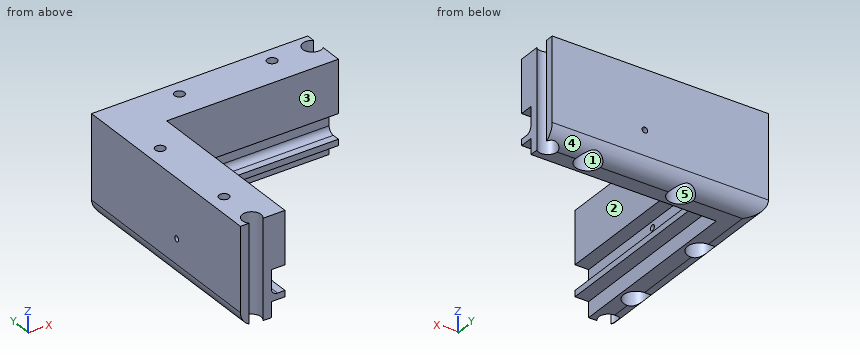
```python
from build123d import *

# Parameters (mm, degrees)
SKETCH2_W           = 18.288
SKETCH2_H           = 40.64
BOSS_EXTRUDE1_DEPTH = 88.9
SKETCH3_W           = 40.64
SKETCH3_H           = 18.288
BOSS_EXTRUDE2_DEPTH = 70.612
SKETCH4_W           = 6.35
SKETCH4_H           = 5.588
SKETCH4_W_2         = 10.16
CUT_EXTRUDE1_DEPTH  = 76.2
SKETCH5_W           = 5.588
SKETCH5_H           = 6.35
SKETCH5_H_2         = 10.16
CUT_EXTRUDE2_DEPTH  = 76.2
SKETCH6_R           = 5.08
CUT_EXTRUDE3_DEPTH  = 15.24
SKETCH7_R           = 2.032
CUT_EXTRUDE4_DEPTH  = 133.128837125
FILLET1_R           = 2.54
FILLET2_R           = 6.35
SKETCH8_R           = 3.81
CUT_EXTRUDE5_DEPTH  = 133.12883729
CUT_EXTRUDE6_REACH  = 125.941
SKETCH9_R           = 1.143
CUT_EXTRUDE7_REACH  = 125.941
SKETCH10_R          = 1.143


with BuildPart() as part:
    # Sketch2 → Boss-Extrude1 (new body)
    with BuildSketch(Plane(origin=(0, 0, 0), x_dir=(1, 0, 0), z_dir=(0, 1, 0))):
        with Locations((9.144, 20.32)):
            Rectangle(SKETCH2_W, SKETCH2_H)
    extrude(amount=BOSS_EXTRUDE1_DEPTH)

    # Sketch3 → Boss-Extrude2 (add)
    with BuildSketch(Plane(origin=(18.288, 0, 0), x_dir=(0, 0, -1), z_dir=(1, 0, 0))):
        with Locations((20.32, 79.756)):
            Rectangle(SKETCH3_W, SKETCH3_H)
    extrude(amount=BOSS_EXTRUDE2_DEPTH)

    # Sketch4 → Cut-Extrude1 (cut)
    with BuildSketch(Plane(origin=(88.9, 0, 0), x_dir=(0, 0, -1), z_dir=(1, 0, 0))):
        with Locations((37.465, 73.406)):
            Rectangle(SKETCH4_W, SKETCH4_H)
        with Locations((26.67, 73.406)):
            Rectangle(SKETCH4_W_2, SKETCH4_H)
    extrude(amount=-CUT_EXTRUDE1_DEPTH, mode=Mode.SUBTRACT)

    # Sketch5 → Cut-Extrude2 (cut)
    with BuildSketch(Plane.XZ):
        with Locations((15.494, -37.465)):
            Rectangle(SKETCH5_W, SKETCH5_H)
        with Locations((15.494, -26.67)):
            Rectangle(SKETCH5_W, SKETCH5_H_2)
    extrude(amount=-CUT_EXTRUDE2_DEPTH, mode=Mode.SUBTRACT)

    # Sketch6 → Cut-Extrude3 (cut)
    with BuildSketch(Plane(origin=(0, 0, -40.64), x_dir=(-1, 0, 0), z_dir=(0, 0, -1))):
        with Locations((-6.35, 19.05)):
            Circle(SKETCH6_R)
        with Locations((-6.35, 57.15)):
            Circle(SKETCH6_R)
        with Locations((-31.75, 82.55)):
            Circle(SKETCH6_R)
        with Locations((-69.85, 82.55)):
            Circle(SKETCH6_R)
    extrude(amount=-CUT_EXTRUDE3_DEPTH, mode=Mode.SUBTRACT)

    # Sketch7 → Cut-Extrude4 (cut, through all)
    with BuildSketch(Plane(origin=(0, 0, -40.64), x_dir=(-1, 0, 0), z_dir=(0, 0, -1))):
        with Locations((-69.85, 82.55)):
            Circle(SKETCH7_R)
        with Locations((-6.35, 57.15)):
            Circle(SKETCH7_R)
        with Locations((-31.75, 82.55)):
            Circle(SKETCH7_R)
        with Locations((-6.35, 19.05)):
            Circle(SKETCH7_R)
    extrude(amount=-CUT_EXTRUDE4_DEPTH, mode=Mode.SUBTRACT)

    # Fillet1
    fillet1_edges = [part.edges().sort_by_distance(p)[0] for p in [
        (12.7, 38.1, -31.75),
        (50.8, 76.2, -31.75),
    ]]
    fillet(fillet1_edges, radius=FILLET1_R)

    # Fillet2
    # the kernel refuses this fillet: 6.35 mm, written as the material it takes off along each edge
    with BuildSketch(Plane(origin=(104.775, 88.9, -40.64), x_dir=(0, -1, 0), z_dir=(-1, 0, 0))) as fillet2_piece_1:
        with BuildLine():
            CenterArc((FILLET2_R, FILLET2_R), FILLET2_R, 180, 90)
            Line((0, FILLET2_R), (0, 0))
            Line((0, 0), (FILLET2_R, 0))
        make_face()
    extrude(amount=120.65, mode=Mode.SUBTRACT)
    with BuildSketch(Plane(origin=(0, -15.875, -40.64), x_dir=(1, 0, 0), z_dir=(0, 1, 0))) as fillet2_piece_2:
        with BuildLine():
            CenterArc((FILLET2_R, -FILLET2_R), FILLET2_R, 90, 90)
            Line((0, -FILLET2_R), (0, 0))
            Line((0, 0), (FILLET2_R, 0))
        make_face()
    extrude(amount=120.65, mode=Mode.SUBTRACT)

    # Sketch8 → Cut-Extrude5 (cut, through all)
    with BuildSketch(Plane.XY):
        with Locations((6.35, 2.54)):
            Circle(SKETCH8_R)
        with Locations((86.36, 82.55)):
            Circle(SKETCH8_R)
    extrude(amount=-CUT_EXTRUDE5_DEPTH, mode=Mode.SUBTRACT)

    # Sketch9 → Cut-Extrude6 (cut, up to next)
    with BuildSketch(Plane.XZ.offset(-76.2), mode=Mode.PRIVATE) as cut_extrude6_sk1:
        with Locations((50.8, -24.13)):
            Circle(SKETCH9_R)
    cut_extrude6_tool1 = extrude(cut_extrude6_sk1.sketch, amount=-CUT_EXTRUDE6_REACH, mode=Mode.PRIVATE) & part.part
    add(cut_extrude6_tool1.solids().sort_by_distance((50.8, 76.2, -24.13))[0], mode=Mode.SUBTRACT)

    # Sketch10 → Cut-Extrude7 (cut, up to next)
    with BuildSketch(Plane(origin=(12.7, 0, 0), x_dir=(0, 0, -1), z_dir=(1, 0, 0)), mode=Mode.PRIVATE) as cut_extrude7_sk1:
        with Locations((24.13, 38.1)):
            Circle(SKETCH10_R)
    cut_extrude7_tool1 = extrude(cut_extrude7_sk1.sketch, amount=-CUT_EXTRUDE7_REACH, mode=Mode.PRIVATE) & part.part
    add(cut_extrude7_tool1.solids().sort_by_distance((12.7, 38.1, -24.13))[0], mode=Mode.SUBTRACT)


solid = part.part
```
Read the model definition and answer for the solid it produces. Units are mm, in the model's axes. Face numbers are marked on the shaded views. A direction names the side the tool comes from. Give positions to 0.01 mm unless a question says otherwise; leave off trailing zeros. Order: outer loops, then holes, each group sorted by start corner. A loop starts at its lowest first (then second) coordinate and runs counter-clockwise, first axis right, second up. Notation, with made-up numbers: (76, 63.5) -> (119, 63.5) arc R10 ccw to (119, 79.5) -> close; hole circle Ø8 at (-39, 54.5). An arc over 180 degrees is marked (long way). Write item = value, one per line.
1. Straight lines are drawn through the part: line 1 along X through (y, z) = (57.15, -32.5); line 2 along Z through (x, y) = (16, 48.5); line 3 along X through (y, z) = (84, -25.5). For each, find the intervals that lie inside material, in ascending order.
Numbers:
line_1 = 0 to 1.27, 11.43 to 18.29
line_2 = -34.29 to -31.75, -21.59 to 0
line_3 = 0 to 26.88, 36.62 to 64.98, 74.72 to 82.84
2. A cutting plane is placed at A-A, the plane z = -24.13. Write down the section's boundary in (x, y), and give its area (3 significant figures).
Numbers:
outline = (0, 0) -> (3.51, 0) arc R3.81 cw (long way) to (9.19, 0) -> (12.7, 0) -> (12.7, 36.96) -> (0, 36.96) -> close; (0, 39.24) -> (12.7, 39.24) -> (12.7, 76.2) -> (49.66, 76.2) -> (49.66, 88.9) -> (0, 88.9) -> close; (51.94, 76.2) -> (88.9, 76.2) -> (88.9, 79.71) arc R3.81 cw (long way) to (88.9, 85.39) -> (88.9, 88.9) -> (51.94, 88.9) -> close; hole circle Ø4.06 at (6.35, 19.05); hole circle Ø4.06 at (6.35, 57.15); hole circle Ø4.06 at (31.75, 82.55); hole circle Ø4.06 at (69.85, 82.55)
area = 1,910 mm²
3. A cutting plane is placed at B-B, the plane y = 57.15. Write down the section's boundary in (x, z), and give its area (3 significant figures).
Numbers:
outline = (0, -34.29) arc R6.35 ccw to (1.27, -38.1) -> (1.27, -25.4) -> (4.32, -25.4) -> (4.32, 0) -> (0, 0) -> close; (8.38, -25.4) -> (11.43, -25.4) -> (11.43, -40.64) -> (12.7, -40.64) -> (12.7, -34.29) -> (18.29, -34.29) -> (18.29, -31.75) -> (15.24, -31.75) arc R2.54 cw to (12.7, -29.21) -> (12.7, -21.59) -> (18.29, -21.59) -> (18.29, 0) -> (8.38, 0) -> close
area = 390 mm²
4. A cutting plane is placed at C-C, the plane x = 50.8. Write down the section's boundary in (y, z), and give its area (3 significant figures).
Numbers:
outline = (70.61, -34.29) -> (76.2, -34.29) -> (76.2, -40.64) -> (82.55, -40.64) arc R6.35 ccw to (88.9, -34.29) -> (88.9, -25.27) -> (76.2, -25.27) -> (76.2, -29.21) arc R2.54 cw to (73.66, -31.75) -> (70.61, -31.75) -> close; (70.61, -21.59) -> (76.2, -21.59) -> (76.2, -22.99) -> (88.9, -22.99) -> (88.9, 0) -> (70.61, 0) -> close
area = 615 mm²
5. A cutting plane is placed at D-D, the plane z = -17. Write down the section's boundary in (x, y), and give its area (3 significant figures).
Numbers:
outline = (0, 0) -> (3.51, 0) arc R3.81 cw (long way) to (9.19, 0) -> (18.29, 0) -> (18.29, 70.61) -> (88.9, 70.61) -> (88.9, 79.71) arc R3.81 cw (long way) to (88.9, 85.39) -> (88.9, 88.9) -> (0, 88.9) -> close; hole circle Ø4.06 at (6.35, 19.05); hole circle Ø4.06 at (6.35, 57.15); hole circle Ø4.06 at (31.75, 82.55); hole circle Ø4.06 at (69.85, 82.55)
area = 2,780 mm²
6. Given pin 1 (11.5 mm diameter, centred on x = 6.35, y = 57.15, fed in from -Z); pin 2 (3 mm diameter, centred on x = 58, z = -33.5, fed in from -Y); pin 3 (3.5 mm diameter, centred on x = 31.75, y = 82.55, fed in from -Z); pin 4 (8 mm diameter, centred on x = 31.5, y = 85, fed in from -Z), each flat-ended and moving along its own axis, determine where each tip first touches the part or whether it passes through.
Numbers:
pin_1 = -40.64
pin_2 = 70.61
pin_3 = through
pin_4 = -39.99
7. The mould has two halves that part along Y. Classify the marked faces 1, 2 and 3: +Y half, -Y half, draft (parallel to the pull), parting line (faces both ways), or undercut.
Numbers:
face_1 = undercut
face_2 = draft
face_3 = -Y half
8. For the marked faces 4 and 5, determine the directions among +Z, -Z, +X, -X, +Y, -Y from which every point of the face is accessible in a straight line to the end or side of a thin tool.
Numbers:
face_4 = -Z, +X, -X, +Y
face_5 = -Z
